Work out the finished part from the listing and answer in its coordinate system (mm). Face numbers are marked on the shaded views. A direction names the side the tool comes from. Give positions to 0.01 mm unless a question says otherwise; leave off trailing zeros. Loops run counter-clockwise (first coordinate to the right, second up) from the corner with the lowest first, then second, coordinate; pieces in that order, holes last. Notation, with made-up numbers: (19, 63) - (55, 63) arc R21 ccw to (55, 90) - close; hole circle Ø6 at (-12.5, -3.75). An arc over 180 degrees is marked (long way). Use CSV: the item, a comma, the result in double quotes.
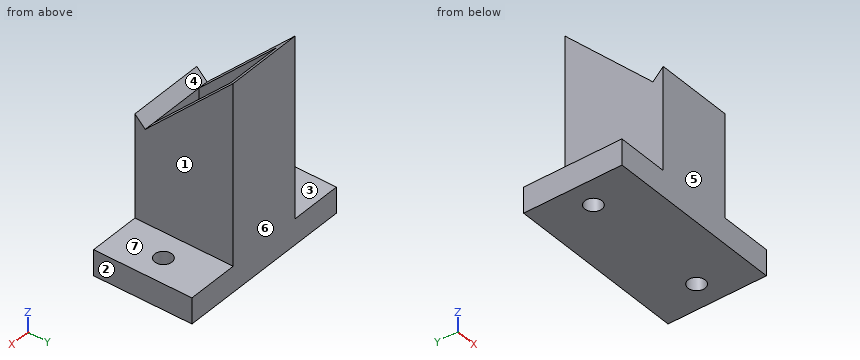
from build123d import *

# Parameters (mm, degrees)
SKETCH1_W             = 15
SKETCH1_H             = 10
BOSS_EXTRUDE1_DEPTH   = 40
CUT_EXTRUDE1_DEPTH    = 40
BOSS_EXTRUDE2_DEPTH   = 15
SKETCH4_W             = 15
SKETCH4_H             = 24.5
BOSS_EXTRUDE3_DEPTH   = 2
SKETCH5_W             = 11
SKETCH5_H             = 15.050743374
CUT_EXTRUDE2_DEPTH    = 44.054307443
SKETCH6_W             = 10
SKETCH6_H             = 19.050743374
SKETCH6_W_2           = 15
SKETCH6_W_3           = 11
SKETCH6_H_2           = 15.050743374
BOSS_EXTRUDE4_DEPTH   = 5
M4X0_7_TAPPED_HOLE1_D = 3.3
M4X0_7_TAPPED_HOLE2_D = 3.3
CUT_EXTRUDE3_DEPTH    = 50.218120539
BOSS_EXTRUDE5_DEPTH   = 15


with BuildPart() as part:
    # Sketch1 → Boss-Extrude1 (new body)
    with BuildSketch(Plane.XY):
        Rectangle(SKETCH1_W, SKETCH1_H)
    extrude(amount=BOSS_EXTRUDE1_DEPTH)

    # Sketch2 → Cut-Extrude1 (cut)
    with BuildSketch(Plane(origin=(7.5, 0, 0), x_dir=(0, 0, -1), z_dir=(1, 0, 0))):
        Polygon((-40, 5), (-40, -5), (-30, -5), align=None)
    extrude(amount=-CUT_EXTRUDE1_DEPTH, mode=Mode.SUBTRACT)

    # Sketch3 → Boss-Extrude2 (add, through all)
    with BuildSketch(Plane.ZY.offset(7.5)):
        Polygon((0, -12.050743374), (0, -5), (30, -5), (25.477447389, -9.522552611), (22.949256626, -12.050743374), align=None)
    extrude(amount=-BOSS_EXTRUDE2_DEPTH)

    # Sketch4 → Boss-Extrude3 (add)
    with BuildSketch(Plane(origin=(0, -12.050743374, 0), x_dir=(-1, 0, 0), z_dir=(0, -1, 0))):
        with Locations((0, -12.25)):
            Rectangle(SKETCH4_W, SKETCH4_H)
    extrude(amount=BOSS_EXTRUDE3_DEPTH)

    # Sketch5 → Cut-Extrude2 (cut, through all)
    with BuildSketch(Plane(origin=(0, 0, 0), x_dir=(-1, 0, 0), z_dir=(0, 0, -1))):
        with Locations((0, -4.525371687)):
            Rectangle(SKETCH5_W, SKETCH5_H)
    extrude(amount=-CUT_EXTRUDE2_DEPTH, mode=Mode.SUBTRACT)

    # Sketch6 → Boss-Extrude4 (add)
    # profile 1 of 4: a face of its own
    with BuildSketch(Plane(origin=(0, 0, 0), x_dir=(-1, 0, 0), z_dir=(0, 0, -1))):
        with Locations((-12.5, -4.525371687)):
            Rectangle(SKETCH6_W, SKETCH6_H)
    # profile 2 of 4: a face of its own
    with BuildSketch(Plane(origin=(0, 0, 0), x_dir=(-1, 0, 0), z_dir=(0, 0, -1))):
        with Locations((12.5, -4.525371687)):
            Rectangle(SKETCH6_W, SKETCH6_H)
    # profile 3 of 4: a face of its own
    with BuildSketch(Plane(origin=(0, 0, 0), x_dir=(-1, 0, 0), z_dir=(0, 0, -1))):
        with Locations((0, -4.525371687)):
            Rectangle(SKETCH6_W_2, SKETCH6_H)
        with Locations((0, -4.525371687)):
            Rectangle(SKETCH6_W_3, SKETCH6_H_2, mode=Mode.SUBTRACT)
    # profile 4 of 4: a face of its own
    with BuildSketch(Plane(origin=(0, 0, 0), x_dir=(-1, 0, 0), z_dir=(0, 0, -1))):
        with Locations((0, -4.525371687)):
            Rectangle(SKETCH6_W_3, SKETCH6_H_2)
    extrude(amount=-BOSS_EXTRUDE4_DEPTH)

    # M4x0.7 Tapped Hole1 (through all)
    with Locations(Plane.XY.offset(5)):
        with Locations((-12.5, -4.525371687)):
            Hole(M4X0_7_TAPPED_HOLE1_D / 2)

    # M4x0.7 Tapped Hole2 (through all)
    with Locations(Plane.XY.offset(5)):
        with Locations((12.5, -4.525371687)):
            Hole(M4X0_7_TAPPED_HOLE2_D / 2)

    # Sketch13 → Cut-Extrude3 (cut, through all)
    with BuildSketch(Plane.ZY.offset(7.5)):
        Polygon((22.949256626, -12.050743374), (24.5, -14.050743374), (24.5, -12.050743374), align=None)
    extrude(amount=-CUT_EXTRUDE3_DEPTH, mode=Mode.SUBTRACT)

    # Sketch14 → Boss-Extrude5 (add)
    with BuildSketch(Plane.ZY.offset(7.5)):
        Polygon((22.949256626, -12.050743374), (22.949256626, -14.050743374), (24.949256626, -14.050743374), align=None)
    extrude(amount=-BOSS_EXTRUDE5_DEPTH)


solid = part.part
Item 1: A cutting plane is placed at C-C on y = 1.5. Determine the outline of the cut face in (x, z).
Determined:
outline,"(-17.5, 0) - (17.5, 0) - (17.5, 5) - (7.5, 5) - (7.5, 36.5) - (5.5, 36.5) - (5.5, 5) - (-5.5, 5) - (-5.5, 36.5) - (-7.5, 36.5) - (-7.5, 5) - (-17.5, 5) - close"
Item 2: A cutting plane is placed at A-A on x = 12.5. Determine the outline of the cut face in (y, z), and give its area (3 significant figures).
Determined:
outline,"(-14.05, 0) - (-6.18, 0) - (-6.18, 5) - (-14.05, 5) - close; (-2.88, 0) - (5, 0) - (5, 5) - (-2.88, 5) - close"
area,"78.8 mm²"
Item 3: The mould has two halves that part along Y. Classify the marked faces 4, 5, 6 and 7: pulls with the +Y half, pulls with the -Y half, needs draft (parallel to the pull), parting line crosses it, or undercut.
Determined:
face 4,"undercut"
face 5,"pulls with the -Y half"
face 6,"pulls with the +Y half"
face 7,"needs draft"
Item 4: A cutting plane is placed at D-D on x = -0.5. Determine the outline of the cut face in (y, z).
Determined:
outline,"(-14.05, 0) - (5, 0) - (5, 40) - (3, 38) - (3, 5) - (-12.05, 5) - (-12.05, 22.95) - (-14.05, 24.95) - close"
Item 5: Find the intervals of material crossed by line 1 (Y direction, x = 12.5, z = 2.75); line 2 (X direction, y = -7, z = 6); line 3 (Y direction, x = 2, z = 8.5), in increasing order.
Determined:
line 1,"y = -14.05 to -6.18, -2.88 to 5"
line 2,"x = -7.5 to -5.5, 5.5 to 7.5"
line 3,"y = -14.05 to -12.05, 3 to 5"
Item 6: For the marked faces 1, 2 and 3, determine the directions among +Z, -Z, +X, -X, +Y, -Y from which every point of the face is accessible in a straight line to the end or side of a thin tool.
Determined:
face 1,"+Z, +X, +Y, -Y"
face 2,"+Z, -Z, +X, +Y, -Y"
face 3,"+Z, -X, +Y, -Y"
Item 7: A cutting plane is placed at B-B on z = 8.5. Determine the outline of the cut face in (x, y).
Determined:
outline,"(-7.5, -14.05) - (7.5, -14.05) - (7.5, 5) - (-7.5, 5) - close; hole (-5.5, -12.05) - (5.5, -12.05) - (5.5, 3) - (-5.5, 3) - close"
Item 8: Given P1, Ø1.5, axis at y = -12, z = 25.5, coming from the +X side; P2, Ø5.5, axis at x = -12.5, y = -4.53, coming from the +Z side; P3, Ø6, axis at y = -2.5, z = 32.5, coming from the +X side; P4, Ø1.5, axis at y = -7.5, z = 6.5, coming from the -X side, each flat-ended and moving along its own axis, determine where each tip first touches the part or whether it passes through.
Determined:
P1,"passes through"
P2,"stops at z = 5"
P3,"stops at x = 7.5"
P4,"stops at x = -7.5"
